from build123d import *

# Parameters (mm, degrees)
BOSS_EXTRUDE1_DEPTH                 = 20
BOSS_EXTRUDE2_DEPTH                 = 20.3
SKETCH4_W                           = 5
SKETCH4_H                           = 15
BOSS_EXTRUDE3_DEPTH                 = 15
CHAMFER2_SIZE                       = 7.5
FILLET1_R                           = 7.5
F_5_5_5_5_DIAMETER_HOLE1_AT_2_COUNT = 2
F_5_5_5_5_DIAMETER_HOLE1_AT_2_PITCH = 12.50000000000005
FILLET2_R                           = 2


with BuildPart() as part:
    # Sketch1 → Boss-Extrude1 (new body)
    with BuildSketch(Plane(origin=(0, 0, 0), x_dir=(0, 0, -1), z_dir=(1, 0, 0))):
        Polygon((-4.59e-15, 15), (-6.12e-15, 20), (-10.000000000000007, 20), (-10.000000000000004, 15), align=None)
        Polygon((4.999999999999994, -20), (6.12e-15, -20), (-6.12e-15, 20), (4.999999999999994, 20), align=None)
    extrude(amount=BOSS_EXTRUDE1_DEPTH)

    # Sketch3 → Boss-Extrude2 (add)
    with BuildSketch(Plane(origin=(20, 0, 0), x_dir=(0, 0, -1), z_dir=(1, 0, 0))):
        Polygon((-10.000000000000007, 20), (-10.000000000000004, 15), (4.999999999999994, 15), (4.999999999999994, 20), align=None)
    extrude(amount=BOSS_EXTRUDE2_DEPTH)

    # Sketch4 → Boss-Extrude3 (add)
    with BuildSketch(Plane(origin=(0, 20, 0), x_dir=(1, 0, 0), z_dir=(0, 1, 0))):
        Polygon((20.00000000000001, -10.000000000000007), (20.000000000000004, 4.999999999999994), (15.000000000000007, 4.999999999999994), (15.000000000000007, -10.000000000000007), align=None)
        with Locations((37.800000000000004, -2.5000000000000067)):
            Rectangle(SKETCH4_W, SKETCH4_H)
    extrude(amount=BOSS_EXTRUDE3_DEPTH)

    # Chamfer2
    chamfer2_edges = [part.edges().sort_by_distance(p)[0] for p in [
        (10, 15, 4.96e-15),
    ]]
    chamfer(chamfer2_edges, length=CHAMFER2_SIZE)

    # Fillet1
    # the kernel refuses this fillet: 7.5 mm, written as the material it adds along each edge
    with BuildSketch(Plane(origin=(0, 15, 7.500000000000005), x_dir=(0, -0.7071067811865472, -0.7071067811865479), z_dir=(1, 0, 0))) as fillet1_piece_1:
        with BuildLine():
            CenterArc((3.068709480812204, -7.500000000000002), FILLET1_R, 90, 40.15544377727605)
            Line((-1.7677669529663684, -1.7677669529663669), (0, 0))
            Line((0, 0), (3.0687094808122044, -1.2e-16))
        make_face()
    extrude(amount=20)
    with BuildSketch(Plane(origin=(20, 15, 26.250000000000007), x_dir=(0, -1, 0), z_dir=(0, 0, -1))) as fillet1_piece_2_section:
        with BuildLine():
            CenterArc((FILLET1_R, -FILLET1_R), FILLET1_R, 90, 90)
            Line((0, -FILLET1_R), (0, 0))
            Line((0, 0), (FILLET1_R, 0))
        make_face()
    fillet1_piece_2 = extrude(amount=31.25, mode=Mode.PRIVATE)
    fillet1_piece_2 = split(fillet1_piece_2, bisect_by=Plane(origin=(20, 24.375, 16.875000000000014), z_dir=(0, 0.7071067811865477, -0.7071067811865474)), keep=Keep.TOP, mode=Mode.PRIVATE)
    add(fillet1_piece_2)
    with BuildSketch(Plane(origin=(20, 15, 26.250000000000007), x_dir=(0, -1, 0), z_dir=(0, 0, -1))) as fillet1_piece_3a_section:
        with BuildLine():
            CenterArc((FILLET1_R, -FILLET1_R), FILLET1_R, 90, 90)
            Line((0, -FILLET1_R), (0, 0))
            Line((0, 0), (FILLET1_R, 0))
        make_face()
    fillet1_piece_3a = extrude(amount=31.25, mode=Mode.PRIVATE)
    fillet1_piece_3a = split(fillet1_piece_3a, bisect_by=Plane(origin=(20, 15.000000000000012, 10), z_dir=(0, 7.1e-16, -1)), keep=Keep.TOP, mode=Mode.PRIVATE)
    fillet1_piece_3a = split(fillet1_piece_3a, bisect_by=Plane(origin=(20, 24.375, 16.87500000000001), z_dir=(0, -0.7071067811865477, 0.7071067811865474)), keep=Keep.TOP, mode=Mode.PRIVATE)
    with BuildSketch(Plane(origin=(0, 15, 7.500000000000005), x_dir=(0, -0.7071067811865472, -0.7071067811865479), z_dir=(1, 0, 0))) as fillet1_piece_3b_section:
        with BuildLine():
            CenterArc((3.068709480812204, -7.500000000000002), FILLET1_R, 90, 40.15544377727605)
            Line((-1.7677669529663684, -1.7677669529663669), (0, 0))
            Line((0, 0), (3.0687094808122044, -1.2e-16))
        make_face()
    fillet1_piece_3b = extrude(amount=27.67177370203051, mode=Mode.PRIVATE)
    fillet1_piece_3b = split(fillet1_piece_3b, bisect_by=Plane(origin=(20, 15, 7.500000000000005), z_dir=(1, 0, 0)), keep=Keep.TOP, mode=Mode.PRIVATE)
    fillet1_piece_3 = fillet1_piece_3a & fillet1_piece_3b
    add(fillet1_piece_3)

    # Sketch7 → Ø4.0 (4) Diameter Hole1 (revolve, cut)
    with BuildSketch(Plane(origin=(15.000000000000007, 27.500000000000004, 2.5000000000000075), x_dir=(0, 0, 1), z_dir=(0, 1, 0))):
        Polygon((0, 0), (-1.22e-15, 5.000000000000001), (1.9999999999999967, 5.000000000000001), (1.9999999999999996, 0.6035533905932753), (2.2500000000000004, -1.73e-15), align=None)
    f_4_0_4_diameter_hole1 = revolve(axis=Axis((8.650000000000016, 27.500000000000004, 2.5000000000000075), (1, 0, 0)), mode=Mode.SUBTRACT)

    # Mirror1: Ø4.0 (4) Diameter Hole1 across plane
    add(f_4_0_4_diameter_hole1.mirror(Plane(origin=(27.65000000000001, 0, -6.4e-15), x_dir=(2.3e-16, 0, 1), z_dir=(1, 0, -2.3e-16))), mode=Mode.SUBTRACT)

    # Sketch9 → Ø5.5 (5.5) Diameter Hole1 (revolve, cut)
    with BuildSketch(Plane(origin=(10, 0, 0), x_dir=(0, -1, 0), z_dir=(1, 0, 0))):
        Polygon((0, 0), (-1.22e-15, 4.999999999999994), (2.749999999999999, 4.999999999999994), (2.7499999999999996, 0.30177669529663986), (2.875, 0), align=None)
    f_5_5_5_5_diameter_hole1 = revolve(axis=Axis((10, 0, 6.349999999999991), (0, 0, -1)), mode=Mode.SUBTRACT)

    # Ø5.5 (5.5) Diameter Hole1 at 2: Ø5.5 (5.5) Diameter Hole1 ×2
    with Locations(*[(0, -i * F_5_5_5_5_DIAMETER_HOLE1_AT_2_PITCH, 0) for i in range(1, F_5_5_5_5_DIAMETER_HOLE1_AT_2_COUNT)]):
        add(f_5_5_5_5_diameter_hole1, mode=Mode.SUBTRACT)

    # Fillet2
    fillet2_edges = [part.edges().sort_by_distance(p)[0] for p in [
        (0, -20, -2.5),
        (20, -20, -2.5),
        (40.3, 15, 2.5000000000000053),
        (17.500000000000007, 35, 10.000000000000007),
        (17.500000000000007, 35, -4.999999999999994),
        (15.000000000000007, 20, 2.500000000000007),
        (37.800000000000004, 35, -4.999999999999994),
        (37.800000000000004, 35, 10.000000000000007),
        (0, 20, 2.500000000000006),
    ]]
    fillet(fillet2_edges, radius=FILLET2_R)


solid = part.part
Verification items for the finished model (mm, model axes). A direction names the side the tool comes from. Round coordinates to 2 decimals unless told otherwise and drop trailing zeros. Order: outer loops, then holes, each group sorted by start corner. A loop starts at its lowest first (then second) coordinate and runs counter-clockwise, first axis right, second up.
1. Release check for a two-part mould opening along Z. For faces 6 (the cylindrical face through (17.771, 29.452, 2.066)), 7 (the cylindrical face through (37.84, 34.4, -4.43)), 8 (the cylindrical face through (37.84, 34.4, 9.43)) record: +Z half, -Z half, draft (parallel to the pull), parting line (faces both ways), or undercut.
Final values:
face 6: undercut
face 7: -Z half
face 8: +Z half
2. Thickness scan on L1, parallel to Y at x = 10, z = -3.3; L2, parallel to X at y = 23, z = -3; L3, parallel to Y at x = 18.05, z = 2.5. Record the ranges inside material, lowest first.
Final values:
L1: y = -20 to -15.25, -9.75 to -2.75, 2.75 to 20
L2: x = 15 to 20, 35.3 to 40.3
L3: y = 10 to 25.5, 29.5 to 35
3. Section check D-D on x = 37.5. Record the cut outline in (y, z).
Final values:
outline: (15, -5) - (33, -5) arc R2 ccw to (35, -3) - (35, 8) arc R2 ccw to (33, 10) - (15, 10) - close; hole circle Ø4 at (27.5, 2.5)
4. Access from +Z, -Z, +X, -X, +Y, -Y to the whole of each face (thin tool, end or side, straight path). Record for faces 1 (the flat face through (20, -6, -3)), 2 (the flat face through (15, 6, -5)), 3 (the flat face through (28, 20, 2)), 4 (the flat face through (40.3, 25.9, 4.3)), 5 (the flat face through (7, 20, 2)).
Final values:
face 1: +Z, -Z, +X, -Y
face 2: -Z, +X, -X, +Y, -Y
face 3: +Z, -Z, +Y
face 4: +Z, -Z, +X, +Y, -Y
face 5: +Z, -Z, -X, +Y
5. Section check A-A on y = 27.5. Record the cut outline in (x, z).
Final values:
outline: (15, -5) - (20, -5) - (20, 0.5) - (15.6, 0.5) - (15, 0.25) - close; (15, 4.75) - (15.6, 4.5) - (20, 4.5) - (20, 10) - (15, 10) - close; (35.3, -5) - (40.3, -5) - (40.3, 0.25) - (39.7, 0.5) - (35.3, 0.5) - close; (35.3, 4.5) - (39.7, 4.5) - (40.3, 4.75) - (40.3, 10) - (35.3, 10) - close
6. Go/stop test with flat-tipped pins: P1, Ø4.5, axis at y = 26.5, z = 5.5, coming from the -X side; P2, Ø6, axis at x = 9, z = -2.5, coming from the +Y side; P3, Ø5, axis at y = -1.5, z = 1, coming from the -X side; P4, Ø3.5, axis at y = 27.5, z = 2.5, coming from the +X side. Record where each tip stops, or that it passes through.
Final values:
P1: stops at x = 15
P2: stops at y = 20
P3: stops at x = 0
P4: passes through
7. Section check C-C on y = 0. Record the cut outline in (x, z) (3 decimals).
Final values:
outline: (0, -5) - (7.25, -5) - (7.25, -0.302) - (7.125, 0) - (0, 0) - close; (12.75, -5) - (20, -5) - (20, 0) - (12.875, 0) - (12.75, -0.302) - close
8. Section check B-B on x = 10. Record the cut outline in (y, z) (3 decimals).
Final values:
outline: (-20, -5) - (-15.25, -5) - (-15.25, -0.302) - (-15.375, 0) - (-20, 0) - close; (-9.75, -5) - (-2.75, -5) - (-2.75, -0.302) - (-2.875, 0) - (-9.625, 0) - (-9.75, -0.302) - close; (2.75, -5) - (20, -5) - (20, 10) - (15, 10) arc R7.5 cw to (12.83, 5.33) - (7.5, 0) - (2.875, 0) - (2.75, -0.302) - close
